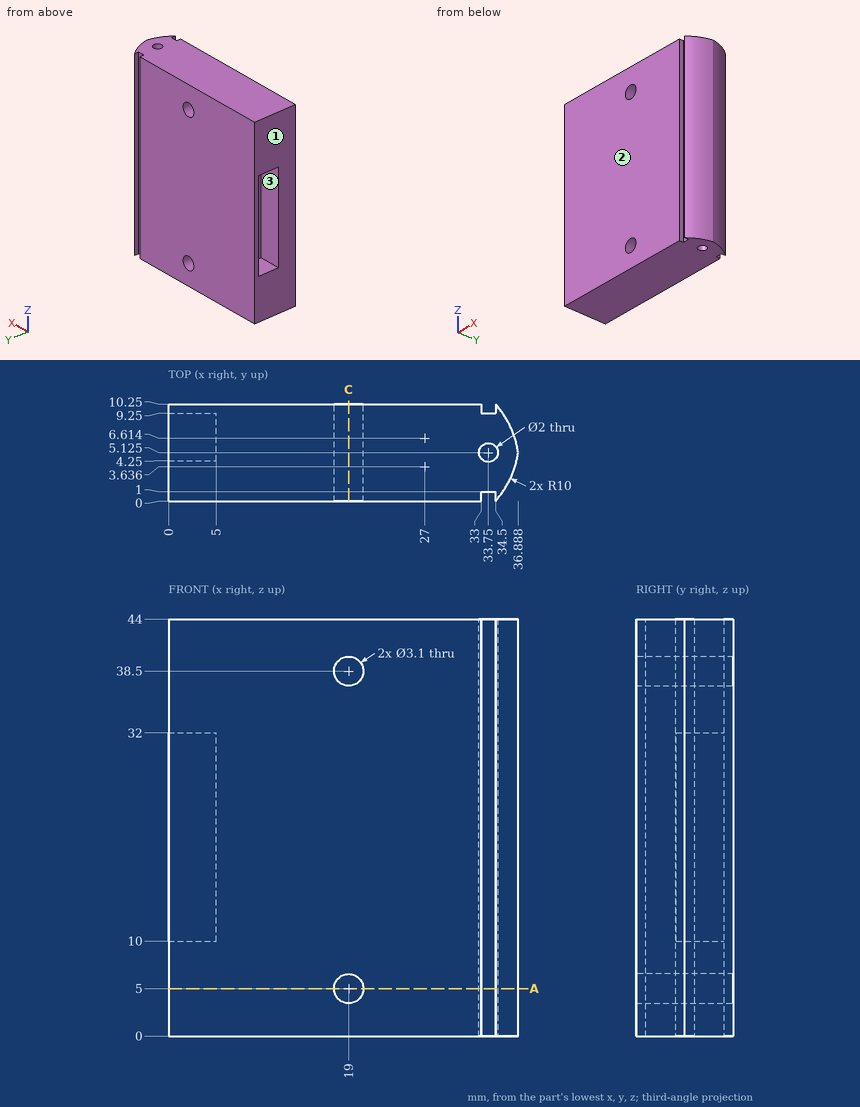
Can you work these out from the drawing? Everything is in mm from the part's minimum corner. Coordinates: 2 decimals unless noted, no trailing zeros. Write each loop counter-clockwise with the first axis right and the second up, starting at its lowest first coordinate (ties: lowest second). Pieces come first, ordered by that corner, then holes. Notation, with made-up numbers: (71.25, 89.25) -> (103.25, 89.25) arc R17 cw to (103.25, 94.25) -> close; hole circle Ø6 at (57, -13). An arc over 180 degrees is marked (long way). Write each question's results on one line, items separated by ' | '. Start each with the question number.
Q1. I'm going to push flat-ended pins straight in: pin 1 (1.1 mm diameter, centred on y = 10, z = 16.5, fed in from -X); pin 2 (3 mm diameter, centred on y = 3.5, z = 26.5, fed in from +X); pin 3 (0.8 mm diameter, centred on y = 9.5, z = 13, fed in from +X) (1 decimal); pin 4 (0.8 mm diameter, centred on x = 34, z = 32, fed in from -Y). Where does each tip first touch, or does it pass through?
Q2. We'd pull the mould along Y, two halves only. Please class the marked faces 1, 2 and 3: +Y half, -Y half, draft (parallel to the pull), parting line (faces both ways), or undercut.
Q3. If I drill on probe 1 along Z at (x, y) = (18.5, 3.5); probe 2 along Y at (x, z) = (33.5, 2.5); probe 3 along X at (y, z) = (6, 20.5) (1 decimal), over which ranges is the centre line in solid material (lowest first)?
Q4. Imagine slicing it at C-C (x = 19). Write out the boundary of the cut face in (y, z).
Q5. Imagine slicing it at A-A (z = 5). State how many separate pieces and enclosed holes the cut face has, then the cut area to 3 significant figures.
Taken from the geometry:
1) pin 1: stops at x = 0 | pin 2: stops at x = 36.87 | pin 3: stops at x = 35.4 | pin 4: stops at y = 1
2) face 1: draft | face 2: -Y half | face 3: undercut
3) probe 1: z = 0 to 3.53, 6.47 to 37.03, 39.97 to 44 | probe 2: y = 1 to 4.16, 6.09 to 9.25 | probe 3: x = 5 to 33.3, 34.2 to 36.7
4) outline: (0, 0) -> (10.25, 0) -> (10.25, 3.45) -> (0, 3.45) -> close; (0, 6.55) -> (10.25, 6.55) -> (10.25, 36.95) -> (0, 36.95) -> close; (0, 40.05) -> (10.25, 40.05) -> (10.25, 44) -> (0, 44) -> close
5) separate pieces: 2 | enclosed holes: 1 | area: 331 mm^2
